Source: CAD feature listing. Evaluate the final solid. Frame: model axes, mm. Face numbers are marked on the shaded views. A direction names the side the tool comes from. Round coordinates to 2 decimals unless told otherwise and drop trailing zeros. Put each result on its own line as item: value. Start each with the question number.
1. Draft query along Y for the marked faces 1, 2 and 3. Return one class per face: pulls with the +Y half, pulls with the -Y half, needs draft (parallel to the pull), parting line crosses it, or undercut.
2. Set-up query: the marked faces 4, 5, 6, 7 and 8. Return all of +Z, -Z, +X, -X, +Y, -Y with unobstructed straight access to the full face (end or side cutting, diameter ignored); none if empty.
3. Contact query for flat-ended pins moving along their axis: pin 1 (21 mm diameter, centred on x = -34, z = 57, fed in from +Y); pin 2 (13 mm diameter, centred on y = 11, z = -89, fed in from -X); pin 3 (1.5 mm diameter, centred on x = 75.5, z = 30, fed in from +Y). Output: stop coordinate, or through.
4. Cut plane A-A (z = -15). State how many separate pieces and enclosed holes the cut face has, then the cut area to 3 significant figures.
5. Material intervals for L1, parallel to Y at x = 88, z = -15; L2, parallel to Z at x = -59, y = 28.5; L3, parallel to Z at x = -74, y = 10, sorted ascending.
```python
from build123d import *

# Parameters (mm, degrees)
ESQUISSE2_W              = 200
ESQUISSE2_H              = 200
BASE_DEPTH               = 35
ESQUISSE3_R              = 15
BLOC_MOTEUR_1_DEPTH      = 80
ESQUISSE4_W              = 10
ESQUISSE4_H              = 22.360679774
ACCES_MOTEUR_DEPTH       = 37
ESQUISSE6_R              = 16.01
BLOC_MOTEUR_2_DEPTH      = 37
ESQUISSE7_R              = 2.5
VIS_MOTEUR_DEPTH         = 146.688022843
ESQUISSE8_R              = 2.5
VIS_PATIN_DEPTH          = 146.688022843
ESQUISSE12_R             = 30
ESPACE_ROUE_DEPTH        = 10
ESQUISSE23_W             = 10
ESQUISSE23_H             = 35
VIDE_TIGE_DEPTH          = 10
VIDE_VIS_REACH           = 219.543
ESQUISSE25_R             = 2.5
VIDE_START               = -1
VIDE_BASE_DEPTH          = 32
BOSS_CROIX_DEPTH         = 4
BOSS_CROIX_DEPTH_BACK    = 2.5
ESQUISSE30_R             = 2
BOSS_VIS_DEPTH           = 35
VIDE_START_2             = -5
ESQUISSE31_R             = 2
VIDE_VIS_COUVERCLE_DEPTH = 5
VIDE_CROIX_DEPTH         = 4


with BuildPart() as part:
    # Esquisse2 → BASE (new body)
    with BuildSketch(Plane(origin=(0, 0, 0), x_dir=(1, 0, 0), z_dir=(0, 1, 0))):
        Rectangle(ESQUISSE2_W, ESQUISSE2_H)
    extrude(amount=BASE_DEPTH)

    # Esquisse3 → BLOC MOTEUR 1. (cut)
    with BuildSketch(Plane(origin=(100, 0, 0), x_dir=(0, 0, -1), z_dir=(1, 0, 0))):
        with Locations((67.5, 10)):
            Circle(ESQUISSE3_R)
    bloc_moteur_1 = extrude(amount=-BLOC_MOTEUR_1_DEPTH, mode=Mode.SUBTRACT)

    # Esquisse4 → ACCES MOTEUR (cut)
    with BuildSketch(Plane.XZ):
        with Locations((25, -67.5)):
            Rectangle(ESQUISSE4_W, ESQUISSE4_H)
    acces_moteur = extrude(amount=-ACCES_MOTEUR_DEPTH, mode=Mode.SUBTRACT)

    # Esquisse6 → BLOC MOTEUR 2 (cut)
    with BuildSketch(Plane(origin=(100, 0, 0), x_dir=(0, 0, -1), z_dir=(1, 0, 0))):
        with Locations((67.5, 10)):
            Circle(ESQUISSE6_R)
    bloc_moteur_2 = extrude(amount=-BLOC_MOTEUR_2_DEPTH, mode=Mode.SUBTRACT)

    # SYM BLOC MOTEUR: BLOC MOTEUR 1., ACCES MOTEUR, BLOC MOTEUR 2 across plane
    add(bloc_moteur_1.mirror(Plane(origin=(0, 0, 0), x_dir=(0, 0, 1), z_dir=(1, 0, 0))), mode=Mode.SUBTRACT)
    add(acces_moteur.mirror(Plane(origin=(0, 0, 0), x_dir=(0, 0, 1), z_dir=(1, 0, 0))), mode=Mode.SUBTRACT)
    add(bloc_moteur_2.mirror(Plane(origin=(0, 0, 0), x_dir=(0, 0, 1), z_dir=(1, 0, 0))), mode=Mode.SUBTRACT)

    # Esquisse7 → VIS MOTEUR (cut, through all)
    with BuildSketch(Plane.XZ):
        with Locations(Location((-76, -27.497129837, 0), (0, 0, 270))):
            Circle(ESQUISSE7_R)
        with Locations(Location((-41.5, -46.319660113, 0), (0, 0, 270))):
            Circle(ESQUISSE7_R)
        with Locations(Location((-41.5, -88.680339887, 0), (0, 0, 270))):
            Circle(ESQUISSE7_R)
        with Locations(Location((-76, -90.002803686, 0), (0, 0, 270))):
            Circle(ESQUISSE7_R)
    vis_moteur = extrude(amount=-VIS_MOTEUR_DEPTH, mode=Mode.SUBTRACT)

    # SYM VIS: VIS MOTEUR across plane
    add(vis_moteur.mirror(Plane(origin=(0, 0, 0), x_dir=(0, 0, 1), z_dir=(1, 0, 0))), mode=Mode.SUBTRACT)

    # Esquisse8 → VIS PATIN (cut, through all)
    with BuildSketch(Plane.XZ):
        with Locations(Location((-55, 77.5, 0), (0, 0, 270))):
            Circle(ESQUISSE8_R)
        with Locations(Location((55, 77.5, 0), (0, 0, 270))):
            Circle(ESQUISSE8_R)
    extrude(amount=-VIS_PATIN_DEPTH, mode=Mode.SUBTRACT)

    # Esquisse12 → ESPACE ROUE (cut)
    with BuildSketch(Plane.ZY.offset(100)):
        with Locations((-67.5, 10)):
            Circle(ESQUISSE12_R)
    espace_roue = extrude(amount=-ESPACE_ROUE_DEPTH, mode=Mode.SUBTRACT)

    # SYM ESPACE ROUE: ESPACE ROUE across plane
    add(espace_roue.mirror(Plane(origin=(0, 0, 0), x_dir=(0, 0, 1), z_dir=(1, 0, 0))), mode=Mode.SUBTRACT)

    # Esquisse23 → VIDE TIGE (cut)
    with BuildSketch(Plane(origin=(100, 0, 0), x_dir=(0, 0, -1), z_dir=(1, 0, 0))):
        with Locations((-90, 17.5)):
            Rectangle(ESQUISSE23_W, ESQUISSE23_H)
        with Locations((15, 17.5)):
            Rectangle(ESQUISSE23_W, ESQUISSE23_H)
    vide_tige = extrude(amount=-VIDE_TIGE_DEPTH, mode=Mode.SUBTRACT)

    # SYM TIGE: VIDE TIGE across plane
    add(vide_tige.mirror(Plane(origin=(0, 0, 0), x_dir=(0, 0, 1), z_dir=(1, 0, 0))), mode=Mode.SUBTRACT)

    # Esquisse25 → VIDE VIS (cut, up to next)
    with BuildSketch(Plane(origin=(90, 0, 0), x_dir=(0, 0, -1), z_dir=(1, 0, 0)), mode=Mode.PRIVATE) as vide_vis_sk1:
        with Locations((-90, 30)):
            Circle(ESQUISSE25_R)
    vide_vis_tool1 = extrude(vide_vis_sk1.sketch, amount=-VIDE_VIS_REACH, mode=Mode.PRIVATE) & part.part
    # Esquisse25 → VIDE VIS (cut, up to next)
    with BuildSketch(Plane(origin=(90, 0, 0), x_dir=(0, 0, -1), z_dir=(1, 0, 0)), mode=Mode.PRIVATE) as vide_vis_sk2:
        with Locations((-90, 20)):
            Circle(ESQUISSE25_R)
    vide_vis_tool2 = extrude(vide_vis_sk2.sketch, amount=-VIDE_VIS_REACH, mode=Mode.PRIVATE) & part.part
    # Esquisse25 → VIDE VIS (cut, up to next)
    with BuildSketch(Plane(origin=(90, 0, 0), x_dir=(0, 0, -1), z_dir=(1, 0, 0)), mode=Mode.PRIVATE) as vide_vis_sk3:
        with Locations((-90, 10)):
            Circle(ESQUISSE25_R)
    vide_vis_tool3 = extrude(vide_vis_sk3.sketch, amount=-VIDE_VIS_REACH, mode=Mode.PRIVATE) & part.part
    # Esquisse25 → VIDE VIS (cut, up to next)
    with BuildSketch(Plane(origin=(90, 0, 0), x_dir=(0, 0, -1), z_dir=(1, 0, 0)), mode=Mode.PRIVATE) as vide_vis_sk4:
        with Locations(Location((15, 10, 0), (0, 0, 180))):
            Circle(ESQUISSE25_R)
    vide_vis_tool4 = extrude(vide_vis_sk4.sketch, amount=-VIDE_VIS_REACH, mode=Mode.PRIVATE) & part.part
    # Esquisse25 → VIDE VIS (cut, up to next)
    with BuildSketch(Plane(origin=(90, 0, 0), x_dir=(0, 0, -1), z_dir=(1, 0, 0)), mode=Mode.PRIVATE) as vide_vis_sk5:
        with Locations(Location((15, 30, 0), (0, 0, 180))):
            Circle(ESQUISSE25_R)
    vide_vis_tool5 = extrude(vide_vis_sk5.sketch, amount=-VIDE_VIS_REACH, mode=Mode.PRIVATE) & part.part
    # Esquisse25 → VIDE VIS (cut, up to next)
    with BuildSketch(Plane(origin=(90, 0, 0), x_dir=(0, 0, -1), z_dir=(1, 0, 0)), mode=Mode.PRIVATE) as vide_vis_sk6:
        with Locations(Location((15, 20, 0), (0, 0, 180))):
            Circle(ESQUISSE25_R)
    vide_vis_tool6 = extrude(vide_vis_sk6.sketch, amount=-VIDE_VIS_REACH, mode=Mode.PRIVATE) & part.part
    add(vide_vis_tool1.solids().sort_by_distance((90, 30, 90))[0], mode=Mode.SUBTRACT)
    add(vide_vis_tool2.solids().sort_by_distance((90, 20, 90))[0], mode=Mode.SUBTRACT)
    add(vide_vis_tool3.solids().sort_by_distance((90, 10, 90))[0], mode=Mode.SUBTRACT)
    add(vide_vis_tool4.solids().sort_by_distance((90, 10, -15))[0], mode=Mode.SUBTRACT)
    add(vide_vis_tool5.solids().sort_by_distance((90, 30, -15))[0], mode=Mode.SUBTRACT)
    add(vide_vis_tool6.solids().sort_by_distance((90, 20, -15))[0], mode=Mode.SUBTRACT)

    # Esquisse27 → VIDE BASE (cut)
    with BuildSketch(Plane(origin=(0, 4, 0), x_dir=(1, 0, 0), z_dir=(0, 1, 0)).offset(VIDE_START)):
        Polygon((-96, -81), (-96, 6), (-86, 6), (-86, 16.142194012), (-86, 50.997196314), (-63, 50.997196314), (-63, 52.319660113), (63, 52.319660113), (63, 50.997196314), (86, 50.997196314), (86, 16.142194012), (86, 6), (96, 6), (96, -81), (86, -81), (86, -96), (-86, -96), (-86, -81), align=None)
        Polygon((-86, 84.002803686), (-63, 84.002803686), (-63, 82.680339887), (63, 82.680339887), (63, 84.002803686), (86, 84.002803686), (86, 96), (-86, 96), align=None)
    extrude(amount=VIDE_BASE_DEPTH, mode=Mode.SUBTRACT)

    # Esquisse29 → BOSS - CROIX (add, two sides: drawn at the far end of the back side and taken through both)
    with BuildSketch(Plane(origin=(0, 4, 0), x_dir=(1, 0, 0), z_dir=(0, 1, 0)).offset(-BOSS_CROIX_DEPTH_BACK)):
        Polygon((-48.536422017, -57.78710173), (-52.983113657, -59.899280259), (-100, -82.232301272), (-100, -85), (-94.173265835, -85), (0, -40.267698728), (94.173265835, -85), (100, -85), (100, -82.232301272), (58.158948273, -62.357801701), (53.712256633, -60.245623173), (5.826734165, -37.5), (100, 7.232301272), (100, 10), (94.173265835, 10), (0, -34.732301272), (-94.173265835, 10), (-100, 10), (-100, 7.232301272), (-5.826734165, -37.5), align=None)
    extrude(amount=BOSS_CROIX_DEPTH + BOSS_CROIX_DEPTH_BACK)

    # Esquisse30 → BOSS VIS (add)
    # profile 1 of 4: a face of its own
    with BuildSketch(Plane(origin=(0, 35, 0), x_dir=(1, 0, 0), z_dir=(0, 1, 0))):
        with BuildLine():
            Line((-5.5, 96), (5.5, 96))
            ThreePointArc((5.5, 96), (0, 90.5), (-5.5, 96))
        make_face()
        with Locations(Location((0, 93.75, 0), (0, 0, 270))):
            Circle(ESQUISSE30_R, mode=Mode.SUBTRACT)
    # profile 2 of 4: a face of its own
    with BuildSketch(Plane(origin=(0, 35, 0), x_dir=(1, 0, 0), z_dir=(0, 1, 0))):
        with BuildLine():
            Line((-5.5, -96), (5.5, -96))
            ThreePointArc((5.5, -96), (0, -90.5), (-5.5, -96))
        make_face()
        with Locations(Location((0, -93.75, 0), (0, 0, 270))):
            Circle(ESQUISSE30_R, mode=Mode.SUBTRACT)
    # profile 3 of 4: a face of its own
    with BuildSketch(Plane(origin=(0, 35, 0), x_dir=(1, 0, 0), z_dir=(0, 1, 0))):
        with BuildLine():
            Line((-96, -27), (-96, -38))
            ThreePointArc((-96, -38), (-90.5, -32.5), (-96, -27))
        make_face()
        with Locations(Location((-93.75, -32.5, 0), (0, 0, 270))):
            Circle(ESQUISSE30_R, mode=Mode.SUBTRACT)
    # profile 4 of 4: a face of its own
    with BuildSketch(Plane(origin=(0, 35, 0), x_dir=(1, 0, 0), z_dir=(0, 1, 0))):
        with BuildLine():
            Line((96, -27), (96, -38))
            ThreePointArc((96, -38), (90.5, -32.5), (96, -27))
        make_face()
        with Locations(Location((93.75, -32.5, 0), (0, 0, 90))):
            Circle(ESQUISSE30_R, mode=Mode.SUBTRACT)
    extrude(amount=-BOSS_VIS_DEPTH)

    # Esquisse31 → VIDE VIS COUVERCLE (cut)
    with BuildSketch(Plane.XZ.offset(VIDE_START_2)):
        with Locations(Location((0, 93.75, 0), (0, 0, 90))):
            Circle(ESQUISSE31_R)
        with Locations(Location((-93.75, 32.5, 0), (0, 0, 90))):
            Circle(ESQUISSE31_R)
        with Locations(Location((0, -93.75, 0), (0, 0, 90))):
            Circle(ESQUISSE31_R)
        with Locations(Location((93.75, 32.5, 0), (0, 0, 270))):
            Circle(ESQUISSE31_R)
    extrude(amount=VIDE_VIS_COUVERCLE_DEPTH, mode=Mode.SUBTRACT)

    # Esquisse36 → VIDE CROIX (cut)
    with BuildSketch(Plane(origin=(0, 4, 0), x_dir=(1, 0, 0), z_dir=(0, 1, 0))):
        Polygon((-95.074987867, -81), (-5.826734165, -38.607079491), (-2.330693666, -40.267698728), (-88.08290687, -81), align=None)
        Polygon((-5.826734165, -36.392920509), (-95.074987867, 6), (-88.08290687, 6), (-2.330693666, -34.732301272), align=None)
        Polygon((88.08290687, -81), (3.248024719, -39.831966478), (7.000943139, -38.049330228), (95.074987867, -81), align=None)
        Polygon((88.08290687, 6), (1.82038942, -34.489906755), (5.57330784, -36.272543005), (95.074987867, 6), align=None)
    extrude(amount=VIDE_CROIX_DEPTH, mode=Mode.SUBTRACT)


solid = part.part
```
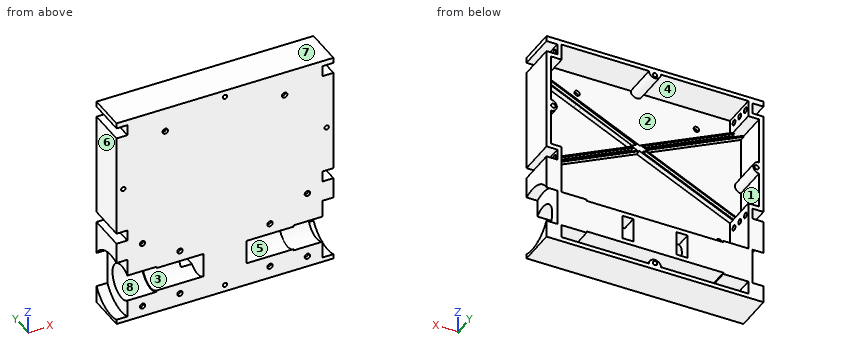
Solution:
1. face 1: needs draft
1. face 2: pulls with the +Y half
1. face 3: undercut
2. face 4: +Y
2. face 5: +X
2. face 6: +Z, -Z, -X, +Y, -Y
2. face 7: +Z, +X, -X, +Y, -Y
2. face 8: -X
3. pin 1: stops at y = 8
3. pin 2: stops at x = -90
3. pin 3: stops at y = 3
4. separate pieces: 7
4. enclosed holes: 0
4. area: 676 mm^2
5. L1: y = 0 to 7.5, 12.5 to 17.5, 22.5 to 27.5, 32.5 to 35
5. L2: z = -100 to -96, -82.68 to -52.32, 96 to 100
5. L3: z = -100 to -96, -84 to -83.51, -51.49 to -51, 96 to 100
